Work out the finished part from the listing and answer in its coordinate system (mm). A direction names the side the tool comes from. Coordinates: 2 decimals unless noted, no trailing zeros. Loops run counter-clockwise (first coordinate to the right, second up) from the corner with the lowest first, then second, coordinate; pieces in that order, holes last. Notation, with made-up numbers: M 79,-1.5 L 84,-1.5 A21 cw 84,26.5 Z; hole C 71.5,-18.75 d2. An arc over 180 degrees is marked long. Write each question's results on one line, items separated by ' | '.
```python
from build123d import *

# Parameters (mm, degrees)
SKETCH3_R          = 4
CUT_EXTRUDE2_DEPTH = 51


with BuildPart() as part:
    # Sketch2 → Revolve1 (revolve)
    with BuildSketch(Plane.XY):
        Polygon((82.5, 0), (56, 0), (56, 6), (24, 6), (24, 20), (31.256462168, 20), (31.256462168, 50), (41.256462168, 50), (41.256462168, 25), (82.5, 25), align=None)
    revolve(axis=Axis((0, 0, 0), (0, 1, 0)))

    # Sketch3 → Cut-Extrude2 (cut, through all)
    with BuildSketch(Plane.XZ):
        with Locations((65, 0)):
            Circle(SKETCH3_R)
        with Locations((45.961940777, -45.961940777)):
            Circle(SKETCH3_R)
        with Locations((0, -65)):
            Circle(SKETCH3_R)
        with Locations((-45.961940777, -45.961940777)):
            Circle(SKETCH3_R)
        with Locations((-65, 0)):
            Circle(SKETCH3_R)
        with Locations((-45.961940777, 45.961940777)):
            Circle(SKETCH3_R)
        with Locations((0, 65)):
            Circle(SKETCH3_R)
        with Locations((45.961940777, 45.961940777)):
            Circle(SKETCH3_R)
    extrude(amount=-CUT_EXTRUDE2_DEPTH, mode=Mode.SUBTRACT)


solid = part.part
```
1) Find section D-D, the plane y = 11. Give the number of separate pieces and of enclosed holes in the cut face, and give its area (3 significant figures).
Check result:
separate pieces: 1 | enclosed holes: 9 | area: 19,200 mm^2
2) Given pin 1 Ø10 at (y, z) = (17.5, 39) entering from +X; pin 2 Ø3 at (x, z) = (-38.5, -10.5) entering from -Y; pin 3 Ø1.5 at (x, z) = (-54, -0.5) entering from +Y, each flat-ended and moving along its own axis, determine where each tip first touches the part or whether it passes through.
Check result:
pin 1: x = 75.17 | pin 2: y = 6 | pin 3: y = 25
3) Find section C-C, the plane y = 30. Give the vertices of the cut face in (x, z).
Check result:
outline: C 0,0 d82.51; hole C 0,0 d62.51
4) Find section A-A, the plane x = -65. Give the vertices of the cut face in (y, z).
Check result:
outline: M 0,-50.81 L 25,-50.81 L 25,-4 L 0,-4 Z; M 0,4 L 25,4 L 25,50.81 L 0,50.81 Z
5) Find section B-B, the plane z = -65. Give the vertices of the cut face in (x, y), and give its area (3 significant figures).
Check result:
outline: M -50.81,0 L -4,0 L -4,25 L -50.81,25 Z; M 4,0 L 50.81,0 L 50.81,25 L 4,25 Z | area: 2,340 mm^2
6) For a pull along X with two mould halves and no side action, classify faces 1 (the face through (17, 0, 54)), 2 (the face through (-61.185, 12.325, 1.201)), 3 (the face through (-17.88, 12.32, 80.54)) as released by +X, released by -X, zero draft, split by the parting line, or undercut.
Check result:
face 1: zero draft | face 2: undercut | face 3: split by the parting line
7) Straight lines are drawn through the part: probe 1 along Y at (x, z) = (-47.5, -34); probe 2 along Z at (x, y) = (14, 4.5); probe 3 along X at (y, z) = (4.5, -66.5). For each, find the intervals that lie inside material, in ascending order. Write a range as [from, to].
Check result:
probe 1: [0, 25] | probe 2: [-81.3, -54.22], [54.22, 81.3] | probe 3: [-48.83, -3.71], [3.71, 48.83]
8) Which of the six approach directions +Z, -Z, +X, -X, +Y, -Y give full straight-line access (tool end or side, diameter ignored) to faces 4 (the face through (51.73, 3.04, 21.45)), 5 (the face through (-49.958, 12.325, 46.138)), 6 (the face through (38, 25, 17))?
Check result:
face 4: -Y | face 5: +Y, -Y | face 6: +Y
